Geometry check sheet. Reference: drawing and pictorial views, mm from the part's lowest x, y, z. A direction names the side the tool comes from. Give positions to 0.01 mm unless a question says otherwise; leave off trailing zeros. Loops run counter-clockwise (first coordinate to the right, second up) from the corner with the lowest first, then second, coordinate; pieces in that order, holes last. Notation, with made-up numbers: (-39.75, 42) - (8.25, 42) arc R26 ccw to (8.25, 73) - close; hole circle Ø4 at (68, -4). An arc over 180 degrees is marked (long way). Answer in a Markdown table with one row per item. Add a question column.
(1) Set-up check for the marked faces 4, 5 and 6: record each of +Z, -Z, +X, -X, +Y, -Y from which the full face is reachable in a straight line by a thin tool's end or side.
(2) Thickness scan on L1, parallel to Z at x = 5.25, y = 24; L2, parallel to Y at x = 14, z = 9.25 (1 decimal); L3, parallel to Y at x = 13.75, z = 12.25 (1 decimal). Record the ranges inside material, lowest first.
(3) Draft check along X on the marked faces 1, 2 and 3. Enter one of: released by +X, released by -X, zero draft, split by the parting line, or undercut.
(4) Sectioned sample at A-A on x = 14. Enter the section's corners in (y, z) (1 decimal), then the cut area to 3 significant figures.
(5) Go/stop test with flat-tipped pins: P1, Ø4.5, axis at y = 25.5, z = 3, coming from the -X side; P2, Ø1.2, axis at x = 2.5, z = 1, coming from the +Y side; P3, Ø10.5, axis at x = 3.5, y = 18, coming from the +Z side. Record where each tip stops, or that it passes through.
(6) Sectioned sample at C-C on y = 9. Enter the section's corners in (x, z).
(7) Sectioned sample at D-D on x = 2.5. Enter the section's corners in (y, z), then the cut area to 3 significant figures.
(8) Sectioned sample at B-B on z = 11.25. Enter the section's corners in (x, y) (1 decimal).
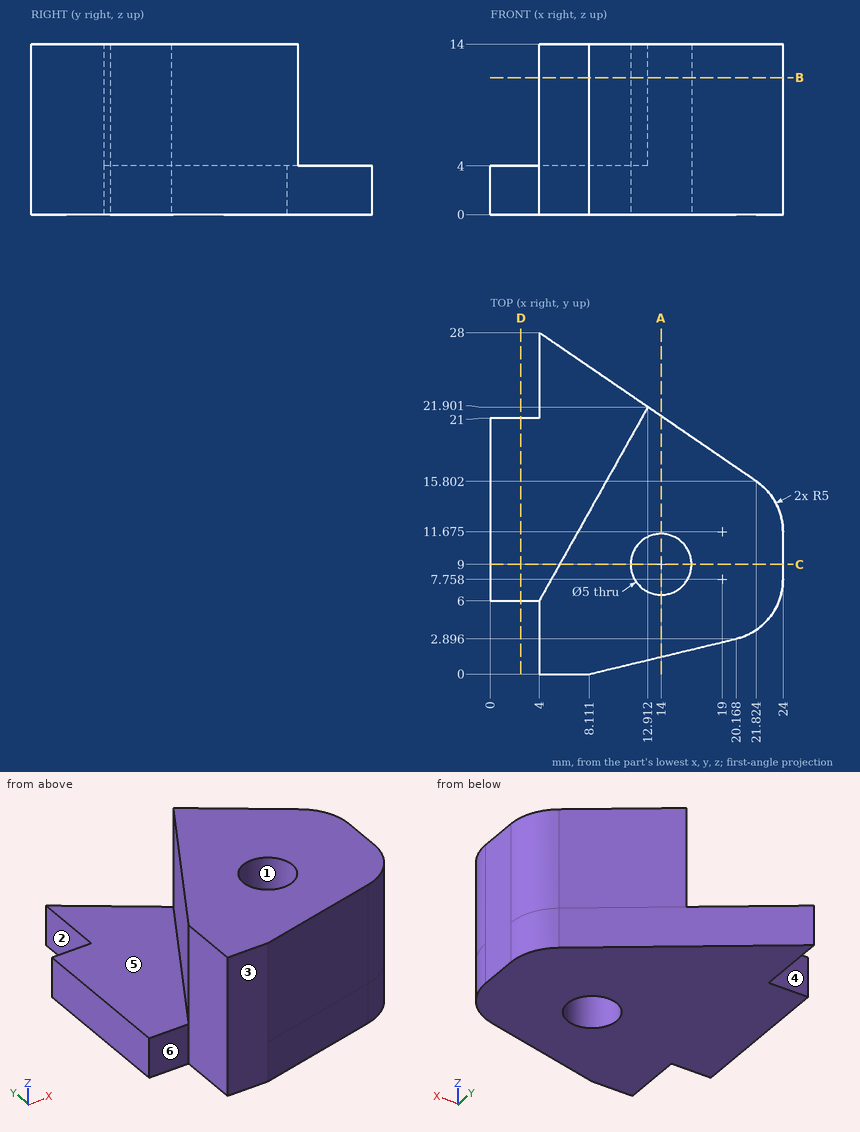
Reply:
| question | item | result |
|---|---|---|
| 1 | face 4 | +Z, -Z, -X, +Y |
| 1 | face 5 | +Z, -X, +Y |
| 1 | face 6 | +Z, -Z, -X, -Y |
| 2 | L1 | 0 to 4 |
| 2 | L2 | 1.4 to 6.5, 11.5 to 21.2 |
| 2 | L3 | 1.4 to 6.5, 11.5 to 21.3 |
| 3 | face 1 | undercut |
| 3 | face 2 | released by -X |
| 3 | face 3 | zero draft |
| 4 | outline | (1.4, 0) - (6.5, 0) - (6.5, 14) - (1.4, 14) - close; (11.5, 0) - (21.2, 0) - (21.2, 14) - (11.5, 14) - close |
| 4 | area | 206 mm^2 |
| 5 | P1 | x = 4 |
| 5 | P2 | y = 21 |
| 5 | P3 | z = 4 |
| 6 | outline | (0, 0) - (11.5, 0) - (11.5, 14) - (5.68, 14) - (5.68, 4) - (0, 4) - close; (16.5, 0) - (24, 0) - (24, 14) - (16.5, 14) - close |
| 7 | outline | (6, 0) - (21, 0) - (21, 4) - (6, 4) - close |
| 7 | area | 60.0 mm^2 |
| 8 | outline | (4, 0) - (8.1, 0) - (20.2, 2.9) arc R5 ccw to (24, 7.8) - (24, 11.7) arc R5 ccw to (21.8, 15.8) - (12.9, 21.9) - (4, 6) - close; hole circle Ø5 at (14, 9) |
